from build123d import *

# Parameters (mm, degrees)
F0_R           = 51.7823878283
F1_DEPTH       = 100
F2_T           = -2.5
F3_R           = 22.1222661474
F3_R_2         = 14.7466183109
F4_DEPTH       = 10
F6_D           = 10
F6_CBORE_D     = 10
F6_CBORE_DEPTH = 5
F7_DEPTH       = 5
F8_DEPTH       = 10


with BuildPart() as f1:
    # F0 (on Front) → F1 (new body)
    with BuildSketch(Plane.XZ):
        Circle(F0_R)
    extrude(amount=F1_DEPTH)

    # F2
    f2_openings = [f1.faces().sort_by_distance(p)[0] for p in [
        (0, -100, 0),
    ]]
    offset(amount=F2_T, openings=f2_openings)

    # F3 (on Front) → F4 (join)
    with BuildSketch(Plane.XZ):
        Circle(F3_R)
        Circle(F3_R_2, mode=Mode.SUBTRACT)
    extrude(amount=F4_DEPTH)

    # F6 (through all)
    with Locations(Plane(origin=(0, 0, 0), x_dir=(1, 0, 0), z_dir=(0, 1, 0))):
        with Locations((0, 0)):
            CounterBoreHole(F6_D / 2, F6_CBORE_D / 2, F6_CBORE_DEPTH)

    # F7 (add): a face of the model
    f7_faces = [f1.faces().sort_by_distance(p)[0] for p in [
        (-50.3177607251, -100, 0),
    ]]
    extrude(f7_faces, amount=F7_DEPTH)

    # F8 (add): a face of the model
    f8_faces = [f1.faces().sort_by_distance(p)[0] for p in [
        (-50.3177607251, -105, 0),
    ]]
    extrude(f8_faces, amount=F8_DEPTH)


solid = f1.part
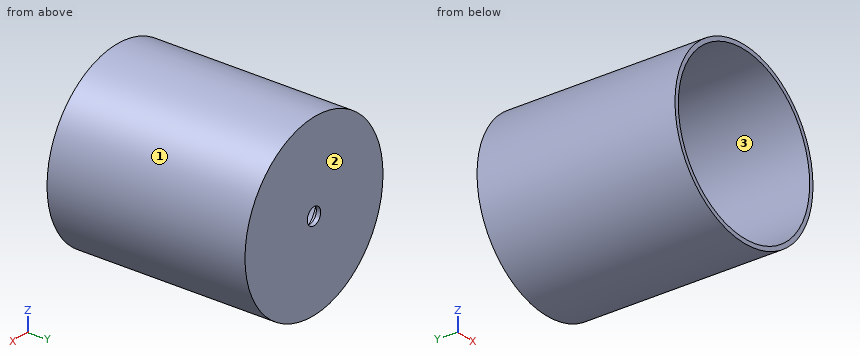
Input: part model. Units: mm. Frame: model coordinates. Face numbers are marked on the shaded views. Coordinates: 2 decimals unless noted, no trailing zeros. Loops run counter-clockwise (first coordinate to the right, second up) from the corner with the lowest first, then second, coordinate; pieces in that order, holes last. Notation, with made-up numbers: (77, 69.25) - (105, 69.25) arc R21 ccw to (105, 95.25) - close; hole circle Ø7 at (70.5, 37). An arc over 180 degrees is marked (long way). Answer in a Markdown table with one row per item. Add a question column.
Item 1: Mould query, pull axis X, two halves, no side actions, for the marked faces 1, 2 and 3. Classes: released by +X, released by -X, zero draft, split by the parting line, or undercut.
Item 2: Section query B-B on x = 0. Return the cut outline in (y, z).
Item 3: Section query D-D on x = -39.5. Return the cut outline in (y, z), then the cut area to 3 significant figures.
Item 4: Contact query for flat-ended pins moving along their axis: P1, Ø17.5, axis at x = 0, z = 0, coming from the +Y side; P2, Ø2, axis at y = -49, z = 34.5, coming from the -X side; P3, Ø2, axis at y = -98.5, z = 22.5, coming from the +X side; P4, Ø2, axis at x = -6, y = -66.5, coming from the +Z side. Output: stop coordinate, or through.
Item 5: Line query: line 1 along Z through (x, y) = (-0.5, -69); line 2 along Z through (x, y) = (0, -8); line 3 along Z through (x, y) = (0, -0.95). Output: solid intervals per line, ascending. Write a range as [from, to].
Item 6: Section query A-A on z = 0. Return the cut outline in (x, y), then the cut area to 3 significant figures.
Item 7: Section query C-C on y = -102.5. Return the cut outline in (x, z).
Recorded:
| question | item | result |
|---|---|---|
| 1 | face 1 | split by the parting line |
| 1 | face 2 | zero draft |
| 1 | face 3 | undercut |
| 2 | outline | (-115, -51.78) - (0, -51.78) - (0, -5) - (-2.5, -5) - (-2.5, -14.75) - (-10, -14.75) - (-10, -22.12) - (-2.5, -22.12) - (-2.5, -49.28) - (-115, -49.28) - close; (-115, 49.28) - (-2.5, 49.28) - (-2.5, 22.12) - (-10, 22.12) - (-10, 14.75) - (-2.5, 14.75) - (-2.5, 5) - (0, 5) - (0, 51.78) - (-115, 51.78) - close |
| 3 | outline | (-115, -33.48) - (0, -33.48) - (0, 33.48) - (-115, 33.48) - (-115, 29.47) - (-2.5, 29.47) - (-2.5, -29.47) - (-115, -29.47) - close |
| 3 | area | 1,070 mm^2 |
| 4 | P1 | y = 0 |
| 4 | P2 | x = -39.49 |
| 4 | P3 | x = 47.11 |
| 4 | P4 | z = 51.54 |
| 5 | line 1 | [-51.78, -49.28], [49.28, 51.78] |
| 5 | line 2 | [-51.78, -49.28], [-22.12, -14.75], [14.75, 22.12], [49.28, 51.78] |
| 5 | line 3 | [-51.78, -5], [5, 51.78] |
| 6 | outline | (-51.78, -115) - (-49.28, -115) - (-49.28, -2.5) - (-22.12, -2.5) - (-22.12, -10) - (-14.75, -10) - (-14.75, -2.5) - (-5, -2.5) - (-5, 0) - (-51.78, 0) - close; (5, -2.5) - (14.75, -2.5) - (14.75, -10) - (22.12, -10) - (22.12, -2.5) - (49.28, -2.5) - (49.28, -115) - (51.78, -115) - (51.78, 0) - (5, 0) - close |
| 6 | area | 907 mm^2 |
| 7 | outline | circle Ø103.56 at (0, 0); hole circle Ø98.56 at (0, 0) |
